from build123d import *

# Parameters (mm, degrees)
SKETCH_1_W      = 20
SKETCH_1_H      = 3
EXTRUDE_1_DEPTH = 3


with BuildPart() as part:
    # 草图1 → 凸台-拉伸1 (new body)
    with BuildSketch(Plane.XY):
        Polygon((50, -53.716238765), (50, -13.716238765), (47, -13.716238765), (47, 26.283761235), (50, 26.283761235), (50, 66.283761235), (47, 66.283761235), (47, 106.283761235), (50, 106.283761235), (50, 146.283761235), (47, 146.283761235), (47, 186.283761235), (50, 186.283761235), (50, 226.283761235), (47, 226.283761235), (47, 266.283761235), (-47, 266.283761235), (-47, 226.283761235), (-50, 226.283761235), (-50, 186.283761235), (-47, 186.283761235), (-47, 146.283761235), (-50, 146.283761235), (-50, 106.283761235), (-47, 106.283761235), (-47, 66.283761235), (-50, 66.283761235), (-50, 26.283761235), (-47, 26.283761235), (-47, -13.716238765), (-50, -13.716238765), (-50, -53.716238765), (-30, -53.716238765), (-30, -50.716238765), (-10, -50.716238765), (-10, -53.716238765), (10, -53.716238765), (10, -50.716238765), (30, -50.716238765), (30, -53.716238765), align=None)
        with Locations((-20, -12.216238765)):
            Rectangle(SKETCH_1_W, SKETCH_1_H, mode=Mode.SUBTRACT)
        with Locations((20, -12.216238765)):
            Rectangle(SKETCH_1_W, SKETCH_1_H, mode=Mode.SUBTRACT)
        with Locations((-20, 174.783761235)):
            Rectangle(SKETCH_1_W, SKETCH_1_H, mode=Mode.SUBTRACT)
        with Locations((20, 174.783761235)):
            Rectangle(SKETCH_1_W, SKETCH_1_H, mode=Mode.SUBTRACT)
        with Locations((-20, 224.783761235)):
            Rectangle(SKETCH_1_W, SKETCH_1_H, mode=Mode.SUBTRACT)
        with Locations((20, 224.783761235)):
            Rectangle(SKETCH_1_W, SKETCH_1_H, mode=Mode.SUBTRACT)
    extrude(amount=EXTRUDE_1_DEPTH)


solid = part.part
Source: CAD feature listing. Evaluate the final solid. Frame: model axes, mm. Give positions to 0.01 mm unless a question says otherwise; leave off trailing zeros. Write each loop counter-clockwise with the first axis right and the second up, starting at its lowest first coordinate (ties: lowest second). Pieces come first, ordered by that corner, then holes. Notation, with made-up numbers: M 85,38.25 L 106,38.25 A18 cw 106,68.25 Z; hole C 26,-30.75 d5. An arc over 180 degrees is marked long. Return JSON: item names as keys, results as strings. Group by question number.
1) Cut plane A-A, the plane z = 2.35. Give the number of separate pieces and of enclosed holes in the cut face, then the cut area to 3 significant figures.
2) Cut plane B-B, the plane y = 103. Output: boundary loops of the cut face in (x, z), then the cut area to 3 significant figures.
3) Ray query, L1, parallel to Y at x = -25, z = 0.35; L2, parallel to X at y = 151.5, z = 2.55. Return the intervals inside material, ascending.
4) First-contact query: pin 1 Ø1.5 at (x, y) = (20.5, 4.5) entering from -Z; pin 2 Ø0.9 at (y, z) = (1.5, 1) entering from -X; pin 3 Ø0.9 at (x, z) = (-25, 1) entering from -Y; pin 4 Ø1.5 at (y, z) = (172.5, 1) entering from +X. Flat tips, straight axial feed; report the tip coordinate or a pass-through.
Data:
{
 "1": {"separate pieces": "1", "enclosed holes": "6", "area": "30,600 mm²"},
 "2": {"outline": "M -47,0 L 47,0 L 47,3 L -47,3 Z", "area": "282 mm²"},
 "3": {"L1": "y = -50.72 to -13.72, -10.72 to 173.28, 176.28 to 223.28, 226.28 to 266.28", "L2": "x = -47 to 47"},
 "4": {"pin 1": "stops at z = 0", "pin 2": "stops at x = -47", "pin 3": "stops at y = -50.72", "pin 4": "stops at x = 47"}
}
